Geometry: final body of the model. Coordinates: model frame, mm. Coordinates: 2 decimals unless noted, no trailing zeros. Order: outer loops, then holes, each group sorted by start corner. A loop starts at its lowest first (then second) coordinate and runs counter-clockwise, first axis right, second up. Notation, with made-up numbers: M 89,65 L 114,65 A13 ccw 114,85 Z; hole C -36,3 d4. An arc over 180 degrees is marked long. Use CSV: the item, a comma, the result in double quotes. Start each with the question number.
1. Section query B-B on x = -34. Return the cut outline in (y, z).
2. Section query A-A on y = 34. Return the cut outline in (x, z), and give its area (3 significant figures).
3. Section query C-C on z = 2.7. Return the cut outline in (x, y), and give its area (3 significant figures).
4. Section query D-D on y = 45. Return the cut outline in (x, z), and give its area (3 significant figures).
5. Material intervals for line 1 (Y direction, x = -34, z = 2.1); line 2 (X direction, y = 34.5, z = 0.5); line 3 (X direction, y = 30, z = 0.2), sorted ascending.
6. Pull-direction query (X, two-part tool) for faces 1 (the flat face through (0, 20, 2)), 2 (the flat face through (-34, 0, 2)), 3 (the cylindrical face through (-32.37, 26.68, 1.97)); classes: pulls with the +X half, pulls with the -X half, needs draft (parallel to the pull), parting line crosses it, or undercut.
from build123d import *

# Parameters (mm, degrees)
SKETCH1_W           = 68
SKETCH1_H           = 50
BOSS_EXTRUDE1_DEPTH = 4
SKETCH4_R           = 7.5
CUT_EXTRUDE1_DEPTH  = 10
FILLET1_R           = 10


with BuildPart() as part:
    # Sketch1 → Boss-Extrude1 (new body)
    with BuildSketch(Plane.XY):
        with Locations((-34, 25)):
            Rectangle(SKETCH1_W, SKETCH1_H)
    extrude(amount=BOSS_EXTRUDE1_DEPTH)

    # Sketch4 → Cut-Extrude1 (cut)
    with BuildSketch(Plane(origin=(0, 0, 0), x_dir=(-1, 0, 0), z_dir=(0, 0, -1))):
        with Locations((34, 34)):
            Circle(SKETCH4_R)
    extrude(amount=-CUT_EXTRUDE1_DEPTH, mode=Mode.SUBTRACT)

    # Fillet1
    fillet1_edges = [part.edges().sort_by_distance(p)[0] for p in [
        (-68, 50, 2),
        (0, 50, 2),
    ]]
    fillet(fillet1_edges, radius=FILLET1_R)


solid = part.part
Results list:
1,outline,"M 0,0 L 26.5,0 L 26.5,4 L 0,4 Z; M 41.5,0 L 50,0 L 50,4 L 41.5,4 Z"
2,outline,"M -68,0 L -41.5,0 L -41.5,4 L -68,4 Z; M -26.5,0 L 0,0 L 0,4 L -26.5,4 Z"
2,area,"212 mm²"
3,outline,"M -68,0 L 0,0 L 0,40 A10 ccw -10,50 L -58,50 A10 ccw -68,40 Z; hole C -34,34 d15"
3,area,"3,180 mm²"
4,outline,"M -66.66,0 L -1.34,0 L -1.34,4 L -66.66,4 Z"
4,area,"261 mm²"
5,line 1,"y = 0 to 26.5, 41.5 to 50"
5,line 2,"x = -68 to -41.48, -26.52 to 0"
5,line 3,"x = -68 to -40.34, -27.66 to 0"
6,face 1,"pulls with the +X half"
6,face 2,"needs draft"
6,face 3,"undercut"
